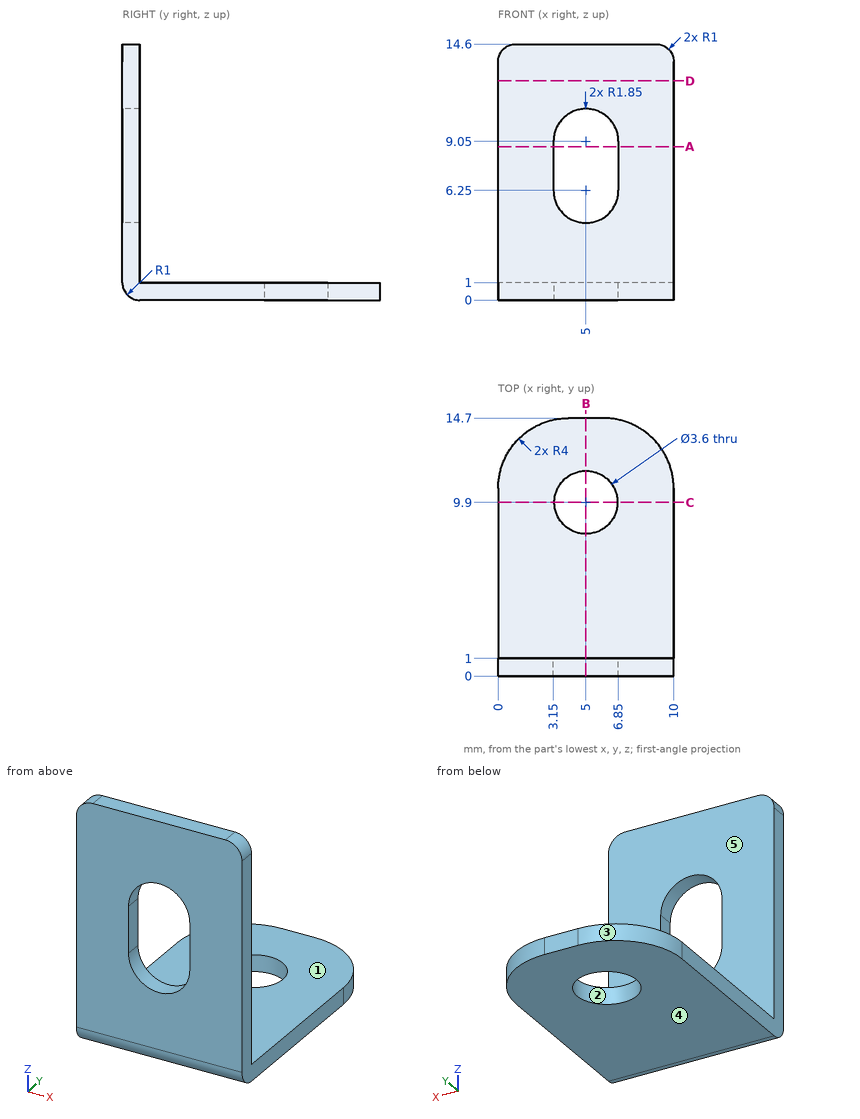
Answer from the drawing. Dimensions are ordinates in mm from the lowest x, y and z of the part. A direction names the side the tool comes from. Round coordinates to 2 decimals unless told otherwise and drop trailing zeros. Loops run counter-clockwise (first coordinate to the right, second up) from the corner with the lowest first, then second, coordinate; pieces in that order, holes last. Notation, with made-up numbers: (53.25, -32.75) - (109.25, -32.75) arc R31 ccw to (109.25, -0.75) - close; hole circle Ø8 at (79.25, 78). An arc over 180 degrees is marked (long way). Return JSON: item names as keys, results as strings. Group by question number.
1. The mould has two halves that part along X. Classify the marked faces 1, 2 and 3: pulls with the +X half, pulls with the -X half, needs draft (parallel to the pull), parting line crosses it, or undercut.
2. Consider probe 1 along Z at (x, y) = (9, 4.5); probe 2 along Y at (x, z) = (5, 0.6). Determine where each line is inside the solid, lowest interval first.
3. Each of these flat-tipped pins is pushed along its axis until it touches: P1, Ø3, axis at x = 6.5, z = 9, coming from the +Y side; P2, Ø5, axis at y = 5.5, z = 8.5, coming from the -X side; P3, Ø4, axis at y = 13, z = 1.5, coming from the +X side; P4, Ø5, axis at x = 5, y = 10.5, coming from the +Z side. Where does it stop, or does it pass through?
4. The part is cut by section B-B on x = 5. Determine the outline of the cut face in (y, z).
5. The part is cut by section A-A on z = 8.75. Determine the outline of the cut face in (x, y), then the cut area to 3 significant figures.
6. Which of the six approach directions +Z, -Z, +X, -X, +Y, -Y give full straight-line access (tool end or side, diameter ignored) to the marked faces 4 and 5?
7. The part is cut by section D-D on z = 12.5. Determine the outline of the cut face in (x, y).
8. The part is cut by section C-C on y = 9.9. Determine the outline of the cut face in (x, z), then the cut area to 3 significant figures.
Resolved:
{
 "1": {"face 1": "needs draft", "face 2": "undercut", "face 3": "pulls with the -X half"},
 "2": {"probe 1": "z = 0 to 1", "probe 2": "y = 0.08 to 8.1, 11.7 to 14.7"},
 "3": {"P1": "stops at y = 1", "P2": "passes through", "P3": "stops at x = 9.98", "P4": "stops at z = 1"},
 "4": {"outline": "(0, 1) arc R1 ccw to (1, 0) - (8.1, 0) - (8.1, 1) - (1, 1) - (1, 4.4) - (0, 4.4) - close; (0, 10.9) - (1, 10.9) - (1, 14.6) - (0, 14.6) - close; (11.7, 0) - (14.7, 0) - (14.7, 1) - (11.7, 1) - close"},
 "5": {"outline": "(0, 0) - (3.15, 0) - (3.15, 1) - (0, 1) - close; (6.85, 0) - (10, 0) - (10, 1) - (6.85, 1) - close", "area": "6.30 mm²"},
 "6": {"face 4": "-Z, +X, -X, +Y, -Y", "face 5": "+Z, +X, -X, +Y"},
 "7": {"outline": "(0, 0) - (10, 0) - (10, 1) - (0, 1) - close"},
 "8": {"outline": "(0, 0) - (3.2, 0) - (3.2, 1) - (0, 1) - close; (6.8, 0) - (10, 0) - (10, 1) - (6.8, 1) - close", "area": "6.40 mm²"}
}
